Study the drawing (mm; zero at the part's minimum x, y, z) and answer. Round coordinates to 2 decimals unless told otherwise and drop trailing zeros. Loops run counter-clockwise (first coordinate to the right, second up) from the corner with the lowest first, then second, coordinate; pieces in that order, holes last. Notation, with made-up numbers: M -35,59.25 L -12,59.25 A26 ccw -12,88.25 Z; hole C -8,-25.5 d2. An arc over 180 degrees is marked long. Put each result on its own line as item: value. Start each with the question number.
(1) Section B-B, the plane y = 44.45 is taken. Determine the outline of the cut face in (x, z).
(2) Flat-ended cylindrical pins translate along their axes: P1, Ø3.5, axis at x = 19.05, z = 4.76, coming from the -Y side; P2, Ø8, axis at x = 62.5, z = 6.5, coming from the +Y side (1 decimal). Find the tip coordinate at first contact, or state that the pin passes through.
(3) Section A-A, the plane x = 38.1 is taken. Determine the outline of the cut face in (y, z), then the cut area to 3 significant figures.
(4) Determine the mould class of the marked faces 1, 2 and 3 for opening direction Y: released by +Y, released by -Y, zero draft, split by the parting line, or undercut.
(5) Section D-D, the plane x = 64.5 is taken. Determine the outline of the cut face in (y, z), then the cut area to 3 significant figures.
(6) Straight lines are drawn through the part: line 1 (Z direction, x = 57, y = 5); line 2 (Y direction, x = 37, z = 18.25); line 3 (X direction, y = 5, z = 6.5) (1 decimal). For each, find the intervals that lie inside material, in ascending order.
(7) Section C-C, the plane z = 14.75 is taken. Determine the outline of the cut face in (x, y).
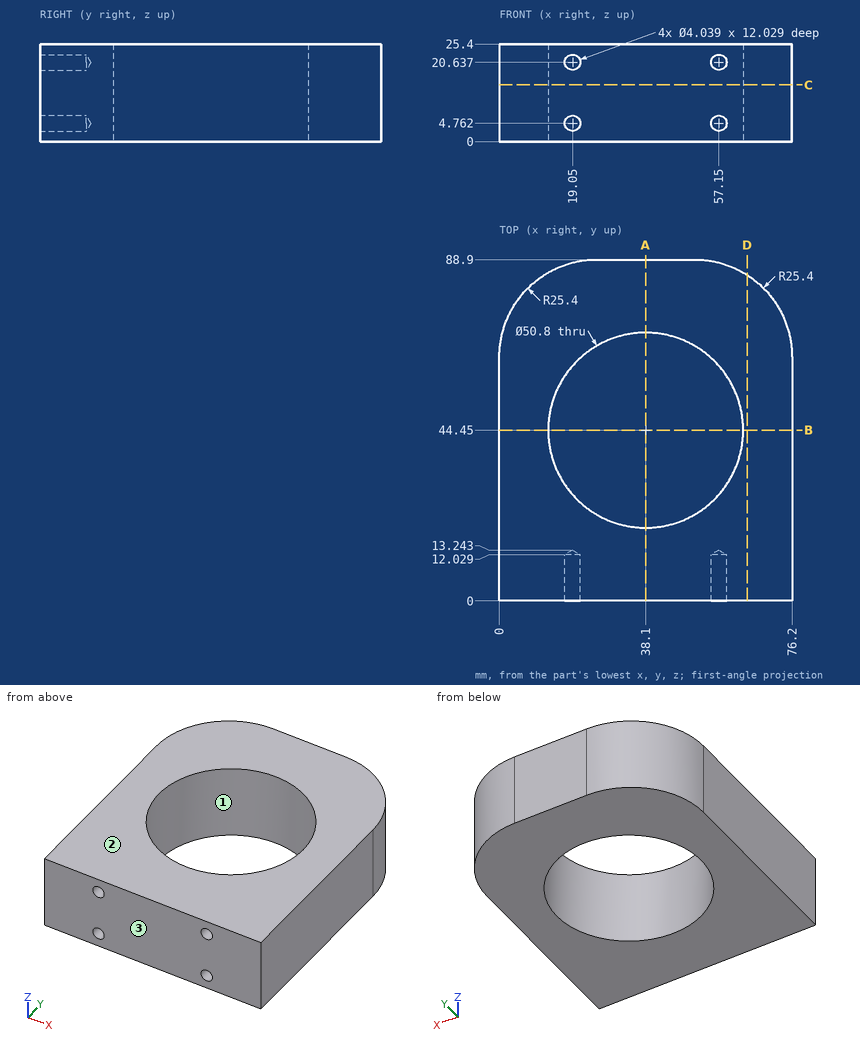
Recorded:
1. outline: M 0,0 L 12.7,0 L 12.7,25.4 L 0,25.4 Z; M 63.5,0 L 76.2,0 L 76.2,25.4 L 63.5,25.4 Z
2. P1: stops at y = 12.19
2. P2: stops at y = 87.7
3. outline: M 0,0 L 19.05,0 L 19.05,25.4 L 0,25.4 Z; M 69.85,0 L 88.9,0 L 88.9,25.4 L 69.85,25.4 Z
3. area: 968 mm²
4. face 1: undercut
4. face 2: zero draft
4. face 3: released by -Y
5. outline: M 0,0 L 84.89,0 L 84.89,25.4 L 0,25.4 Z
5. area: 2,160 mm²
6. line 1: z = 0 to 2.75, 6.78 to 18.62, 22.65 to 25.4
6. line 2: y = 0 to 19.07, 69.83 to 88.9
6. line 3: x = 0 to 18, 20.1 to 56.1, 58.2 to 76.2
7. outline: M 0,0 L 76.2,0 L 76.2,63.5 A25.4 ccw 50.8,88.9 L 25.4,88.9 A25.4 ccw 0,63.5 Z; hole C 38.1,44.45 d50.8
